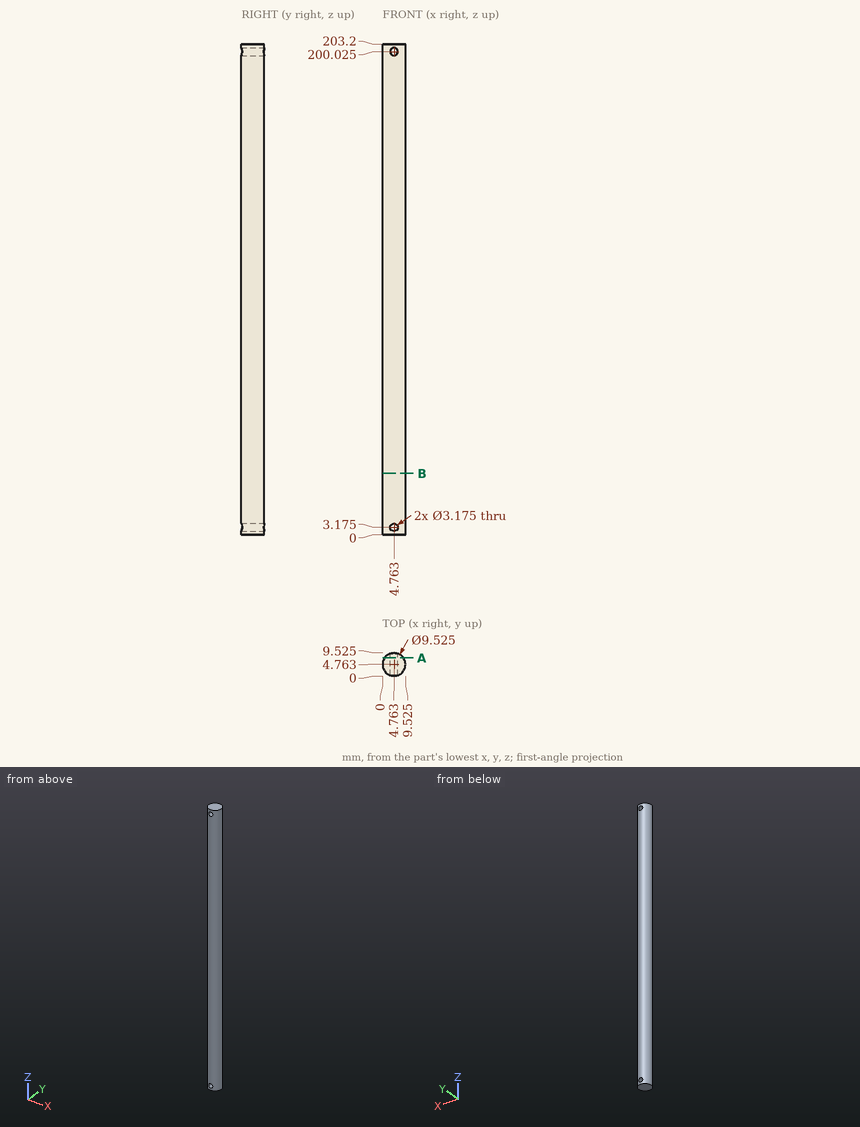
Geometry: see drawing. Coordinates: mm, zero at the bounding-box minimum. Give positions to 0.01 mm unless a question says otherwise; leave off trailing zeros. Loops run counter-clockwise (first coordinate to the right, second up) from the corner with the lowest first, then second, coordinate; pieces in that order, holes last. Notation, with made-up numbers: (-10, -39.75) - (47, -39.75) arc R6 ccw to (47, -30.75) - close; hole circle Ø1 at (5.25, -23.5). An arc over 180 degrees is marked (long way). One line per question, with ' | ' between items. Start each with the question number.
(1) Section query B-B on z = 25.5. Return loops of the section in (x, y) (1 decimal).
(2) Section query A-A on y = 7.5. Return loops of the section in (x, z) (1 decimal), then the cut area to 3 significant figures.
(3) Contact query for flat-ended pins moving along their axis: pin 1 (5 mm diameter, centred on y = 4, z = 24, fed in from -X); pin 2 (4 mm diameter, centred on x = 1.5, z = 134.5, fed in from -Y); pin 3 (2 mm diameter, centred on y = 2, z = 76, fed in from +X); pin 4 (1.5 mm diameter, centred on y = 8, z = 30, fed in from -X). Output: stop coordinate, or through.
(4) Ray query, line 1 (Z direction, x = 4.5, y = 1.75); line 2 (Z direction, x = 4.75, y = 5); line 3 (X direction, y = 5, z = 169) (1 decimal). Return the intervals inside material, ascending. Write a range as from..to.
The answers:
1) outline: circle Ø9.5 at (4.8, 4.8)
2) outline: (0.9, 0) - (8.7, 0) - (8.7, 203.2) - (0.9, 203.2) - close; hole circle Ø3.2 at (4.8, 3.2); hole circle Ø3.2 at (4.8, 200) | area: 1,570 mm2
3) pin 1: x = 0 | pin 2: y = 0.17 | pin 3: x = 9.19 | pin 4: x = 0.7
4) line 1: 0..1.61, 4.74..198.46, 201.59..203.2 | line 2: 0..1.59, 4.76..198.44, 201.61..203.2 | line 3: 0..9.5
